Geometry check sheet. Reference: the model listing, model coordinates, mm. A direction names the side the tool comes from. Give positions to 0.01 mm unless a question says otherwise; leave off trailing zeros. Write item = value, one per line.
```python
from build123d import *

# Parameters (mm, degrees)
F2_ANGLE = 338
F3_R     = 43
F3_R_2   = 23
F4_DEPTH = 25


with BuildPart() as f2:
    # F1 (on Right) → F2 (revolve)
    with BuildSketch(Plane.YZ):
        Polygon((-14.592193, 16.6), (-13.878119, 17.1), (-13.878119, 26.85), (-14.878119, 26.85), (-21.628119, 20.1), (-21.628119, 17.1), (-17.448489, 17.1), (-17.448489, 16.6), (-16.734415, 17.1), (-16.734415, 16.6), (-16.020341, 17.1), (-16.020341, 16.6), (-15.306267, 17.1), (-15.306267, 16.6), (-14.592193, 17.1), align=None)
    revolve(axis=Axis((0, -8.217514, 0), (0, 1, 0)), revolution_arc=F2_ANGLE)

    # F3 (on Front) → F4 (cut)
    with BuildSketch(Plane.XZ):
        Circle(F3_R)
        Circle(F3_R_2, mode=Mode.SUBTRACT)
    extrude(amount=F4_DEPTH, mode=Mode.SUBTRACT)

    # F5 (on face) → F6 (revolve, cut)
    with BuildSketch(Plane(origin=(0, 0, 0), x_dir=(0, 1, 0), z_dir=(0.927184, 0, 0.374607))):
        Polygon((-15.378119, 18.1), (-15.378119, 21.5), (-18.106798, 21.5), (-19.910035, 19.696764), (-18.313271, 18.1), align=None)
    revolve(axis=Axis((0, -8.217514, 0), (0, 1, 0)), mode=Mode.SUBTRACT)


solid = f2.part
```
Item 1: Tool access check on faces 4 (the cylindrical face through (3.953, -19.509, -16.637)), 5 (the flat face through (17, -13.878, 4)), 6 (the flat face through (-7.967, -18.668, 19.718)), 7 (the conical face through (3.87, -17.245, -16.289)). Record the directions out of +Z, -Z, +X, -X, +Y, -Y that give a thin tool (end or side, any length) a straight path to the whole face; none if there is none.
Answer:
face_4 = -Y
face_5 = +Z, -Z, +X, -X, +Y
face_6 = +Z, +Y, -Y
face_7 = none
Item 2: Draft check along Y on faces 1 (the conical face through (4.68, -21.49, -19.69)), 2 (the cylindrical face through (3.45, -16.27, -22.74)), 3 (the conical face through (4.2, -18.6, -17.9)). Enter one of: +Y half, -Y half, draft (parallel to the pull), parting line (faces both ways), or undercut.
Answer:
face_1 = -Y half
face_2 = draft
face_3 = undercut
Item 3: Gauge pin test, flat ends, axial feed: pin 1 (2 mm diameter, centred on x = 7.5, y = -18.5, fed in from +Z); pin 2 (21.5 mm diameter, centred on x = -4, z = -9, fed in from -Y); pin 3 (1.5 mm diameter, centred on y = -17.5, z = 10, fed in from -X); pin 4 (1 mm diameter, centred on y = -19.5, z = -6, fed in from -X). Record the tip position at first contact, or that the pin passes through.
Answer:
pin_1 = 22.06
pin_2 = -21.63
pin_3 = -21.06
pin_4 = -21.94
Item 4: Thickness scan on L1, parallel to X at y = -17.5, z = 0.5; L2, parallel to Z at x = -8, y = -18.5; L3, parallel to Z at x = -11.5, y = -19.75. Record the ranges inside material, lowest first. Write a range as [from, to].
Answer:
L1 = [-22.99, -21.49], [-18.09, -17.09], [17.09, 18.09], [21.49, 22.99]
L2 = [-21.56, -19.53], [-16.44, -15.11], [15.11, 16.44], [19.53, 19.8]
L3 = [-18.73, -16.19], [-15.79, -12.66], [12.66, 15.79], [16.19, 18.73]
Item 5: Section check A-A, the plane z = 0. Give the number of separate pieces and of enclosed holes in the cut face, plus the area to 3 significant figures.
Answer:
separate_pieces = 2
enclosed_holes = 2
area = 59.8 mm^2
